Geometry: see drawing. Coordinates: mm, zero at the bounding-box minimum. A direction names the side the tool comes from. Round coordinates to 2 decimals unless told otherwise and drop trailing zeros. Write each loop counter-clockwise with the first axis right and the second up, starting at its lowest first coordinate (ties: lowest second). Pieces come first, ordered by that corner, then holes. Notation, with made-up numbers: M 62,50.25 L 112,50.25 A9 cw 112,62.25 Z; hole C 27,-14 d8. An arc over 180 degrees is marked long. Write each question's results on one line, items separated by ' | '. Start each with the question number.
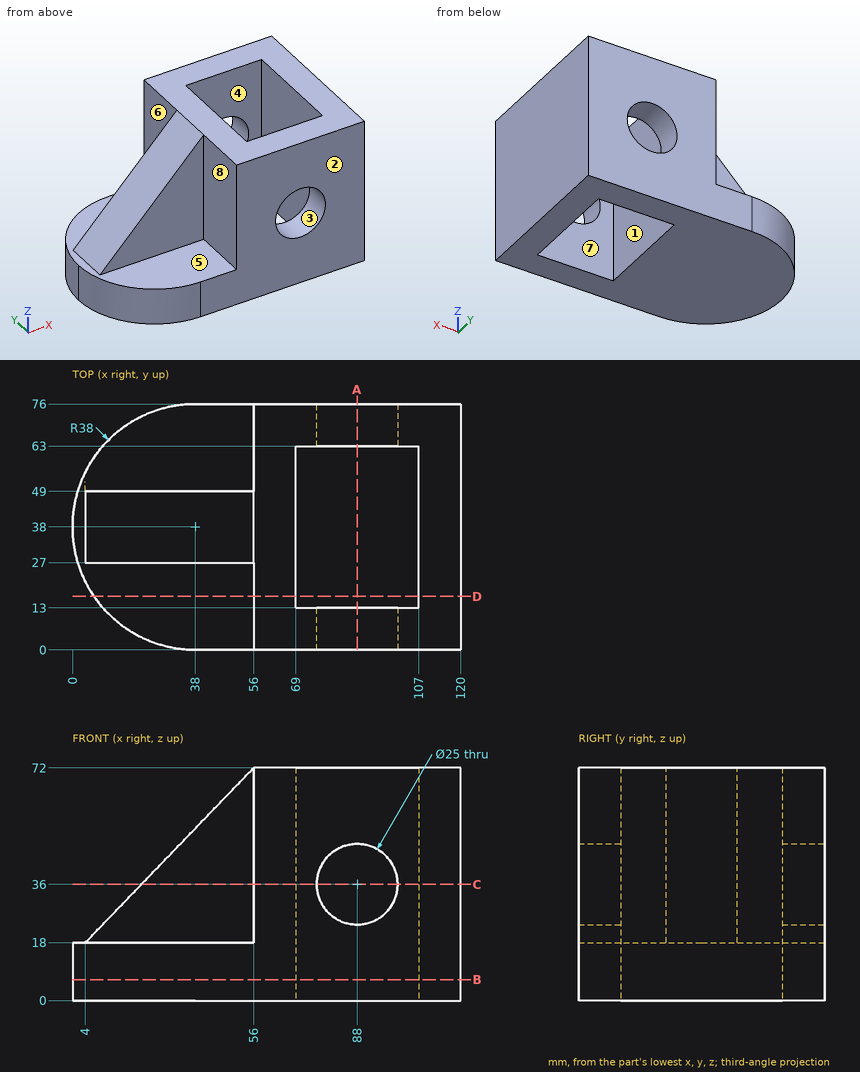
1. Cut plane A-A on x = 88. Output: boundary loops of the cut face in (y, z), and give its area (3 significant figures).
2. Access query for the marked faces 5, 6, 7 and 8. Directions: +Z, -Z, +X, -X, +Y, -Y. A direction counts if a zero-diameter tool reaches every point of the face in a straight line with its end or side. Return the directions, or none.
3. Cut plane B-B on z = 6.5. Output: boundary loops of the cut face in (x, y).
4. Cut plane D-D on y = 16.5. Output: boundary loops of the cut face in (x, z).
5. Line query: L1, parallel to X at y = 51, z = 31; L2, parallel to Y at x = 93.5, z = 60; L3, parallel to X at y = 68, z = 36. Output: solid intervals per line, ascending. Write a range as from..to.
6. Draft query along Y for the marked faces 1, 2, 3 and 4. Return one class per face: +Y half, -Y half, draft (parallel to the pull), parting line (faces both ways), or undercut.
7. Cut plane C-C on z = 36. Output: boundary loops of the cut face in (x, y), and give its area (3 significant figures).
8. Contact query for flat-ended pins moving along their axis: P1, Ø17, axis at x = 28.5, y = 40, coming from the +Z side; P2, Ø13.5, axis at y = 20, z = 50.5, coming from the -X side; P3, Ø5, axis at y = 42, z = 14.5, coming from the -X side; P4, Ø15, axis at x = 88, z = 36, coming from the +Y side. Output: stop coordinate, or through.
Answers follow:
1) outline: M 0,0 L 13,0 L 13,23.5 L 0,23.5 Z; M 0,48.5 L 13,48.5 L 13,72 L 0,72 Z; M 63,0 L 76,0 L 76,23.5 L 63,23.5 Z; M 63,48.5 L 76,48.5 L 76,72 L 63,72 Z | area: 1,220 mm2
2) face 5: +Z, -X | face 6: +Z, -X, +Y | face 7: +Z, -Z | face 8: +Z, -X, -Y
3) outline: M 0,38 A38 ccw 38,0 L 120,0 L 120,76 L 38,76 A38 ccw Z; hole M 69,13 L 107,13 L 107,63 L 69,63 Z
4) outline: M 6.67,0 L 69,0 L 69,72 L 56,72 L 56,18 L 6.67,18 Z; M 107,0 L 120,0 L 120,72 L 107,72 Z
5) L1: x = 56..69, 107..120 | L2: y = 0..13, 63..76 | L3: x = 56..75.5, 100.5..120
6) face 1: undercut | face 2: -Y half | face 3: draft | face 4: undercut
7) outline: M 21.33,27 L 56,27 L 56,0 L 75.5,0 L 75.5,13 L 69,13 L 69,63 L 75.5,63 L 75.5,76 L 56,76 L 56,49 L 21.33,49 Z; M 100.5,0 L 120,0 L 120,76 L 100.5,76 L 100.5,63 L 107,63 L 107,13 L 100.5,13 Z | area: 3,080 mm2
8) P1: stops at z = 52.27 | P2: stops at x = 56 | P3: stops at x = 0.03 | P4: passes through
